Design review of the part built by this model. Coordinates are the model's own, in mm. A direction names the side the tool comes from. Round coordinates to 2 decimals unless told otherwise and drop trailing zeros. Return JSON: item names as keys, results as strings. Group by question number.
(1) We need section A-A, the plane z = 2.05. Give the number of separate pieces and of enclosed holes in the cut face, and give its area (3 significant figures).
(2) For faces 1 (the flat face through (2.533, -12.053, 1.479)), 2 (the flat face through (-2.533, 12.053, 1.479)), 3 (the cylindrical face through (-8.21, -8.05, 1.48)), 4 (the cylindrical face through (-11.13, 9.53, 1.48)), list the 3-axis set-ups (+Z, -Z, +X, -X, +Y, -Y) from which the entire face can be reached by the end or side of a thin tool; tool diameter is ignored.
(3) The part is to be moulded in two halves that separate along Y. For faces 5 (the cylindrical face through (6.02, -9.8, 1.48)), 6 (the cylindrical face through (8.636, 13.469, 1.479)), 7 (the flat face through (-5.354, -11.117, 1.479)), say which applies: pulls with the +Y half, pulls with the -Y half, needs draft (parallel to the pull), parting line crosses it, or undercut.
(4) Clearance check with flat-ended pins moving along their axes: pin 1 (1.3 mm diameter, centred on y = -12.5, z = 1.5, fed in from +X); pin 2 (1.3 mm diameter, centred on y = 12.5, z = 1.5, fed in from -X). State where each tip first meets the part, or that it passes through.
(5) Wall thickness on L1, parallel to X at y = -12, z = 1.5; L2, parallel to Y at x = 13.5, z = 1.4; L3, parallel to X at y = 13, z = 2.45: over which ranges is each line inside the solid? List them lowest first. Write a range as [from, to].
from build123d import *

# Parameters (mm, degrees)
BOSS_EXTRU_1_DEPTH           = 3
R_P_TITION_CIRCULAIRE2_COUNT = 14
ESQUISSE5_R                  = 11.5
BOSS_EXTRU_2_DEPTH           = 3
ESQUISSE6_R                  = 3
ESQUISSE6_R_2                = 1.75
ENL_V_MAT_EXTRU_1_DEPTH      = 4


with BuildPart() as part:
    # Esquisse4 → Boss.-Extru.1 (new body)
    with BuildSketch(Plane.XY):
        with BuildLine():
            Line((0, 13.155696691), (0, 11.5))
            ThreePointArc((0, 11.5), (1.385979557, 11.416175396), (2.751754038, 11.165923594))
            Line((2.751754038, 11.165923594), (3.147934042, 12.773522094))
            ThreePointArc((3.147934042, 12.773522094), (3.010357566, 14.324173734), (2.517223611, 15.800746352))
            ThreePointArc((2.517223611, 15.800746352), (1.928319383, 15.883374464), (1.336751397, 15.944061456))
            ThreePointArc((1.336751397, 15.944061456), (0.504624377, 14.628382005), (0, 13.155696691))
        make_face()
    extrude(amount=BOSS_EXTRU_1_DEPTH)


with BuildPart() as r_p_tition_circulaire2_1:
    # R_p_tition circulaire2: pattern copy
    add(part.part.rotate(Axis((0, 0, 0), (0, 0, 1)), 1 * 360 / R_P_TITION_CIRCULAIRE2_COUNT))


with BuildPart() as r_p_tition_circulaire2_2:
    # R_p_tition circulaire2: pattern copy
    add(part.part.rotate(Axis((0, 0, 0), (0, 0, 1)), 2 * 360 / R_P_TITION_CIRCULAIRE2_COUNT))


with BuildPart() as r_p_tition_circulaire2_3:
    # R_p_tition circulaire2: pattern copy
    add(part.part.rotate(Axis((0, 0, 0), (0, 0, 1)), 3 * 360 / R_P_TITION_CIRCULAIRE2_COUNT))


with BuildPart() as r_p_tition_circulaire2_4:
    # R_p_tition circulaire2: pattern copy
    add(part.part.rotate(Axis((0, 0, 0), (0, 0, 1)), 4 * 360 / R_P_TITION_CIRCULAIRE2_COUNT))


with BuildPart() as r_p_tition_circulaire2_5:
    # R_p_tition circulaire2: pattern copy
    add(part.part.rotate(Axis((0, 0, 0), (0, 0, 1)), 5 * 360 / R_P_TITION_CIRCULAIRE2_COUNT))


with BuildPart() as r_p_tition_circulaire2_6:
    # R_p_tition circulaire2: pattern copy
    add(part.part.rotate(Axis((0, 0, 0), (0, 0, 1)), 6 * 360 / R_P_TITION_CIRCULAIRE2_COUNT))


with BuildPart() as r_p_tition_circulaire2_7:
    # R_p_tition circulaire2: pattern copy
    add(part.part.rotate(Axis((0, 0, 0), (0, 0, 1)), 7 * 360 / R_P_TITION_CIRCULAIRE2_COUNT))


with BuildPart() as r_p_tition_circulaire2_8:
    # R_p_tition circulaire2: pattern copy
    add(part.part.rotate(Axis((0, 0, 0), (0, 0, 1)), 8 * 360 / R_P_TITION_CIRCULAIRE2_COUNT))


with BuildPart() as r_p_tition_circulaire2_9:
    # R_p_tition circulaire2: pattern copy
    add(part.part.rotate(Axis((0, 0, 0), (0, 0, 1)), 9 * 360 / R_P_TITION_CIRCULAIRE2_COUNT))


with BuildPart() as r_p_tition_circulaire2_10:
    # R_p_tition circulaire2: pattern copy
    add(part.part.rotate(Axis((0, 0, 0), (0, 0, 1)), 10 * 360 / R_P_TITION_CIRCULAIRE2_COUNT))


with BuildPart() as r_p_tition_circulaire2_11:
    # R_p_tition circulaire2: pattern copy
    add(part.part.rotate(Axis((0, 0, 0), (0, 0, 1)), 11 * 360 / R_P_TITION_CIRCULAIRE2_COUNT))


with BuildPart() as r_p_tition_circulaire2_12:
    # R_p_tition circulaire2: pattern copy
    add(part.part.rotate(Axis((0, 0, 0), (0, 0, 1)), 12 * 360 / R_P_TITION_CIRCULAIRE2_COUNT))


with BuildPart() as r_p_tition_circulaire2_13:
    # R_p_tition circulaire2: pattern copy
    add(part.part.rotate(Axis((0, 0, 0), (0, 0, 1)), 13 * 360 / R_P_TITION_CIRCULAIRE2_COUNT))


with BuildPart() as part_1:
    add(part.part)

    add(r_p_tition_circulaire2_1.part)  # Boss.-Extru.2 merges R_p_tition circulaire2_1

    add(r_p_tition_circulaire2_2.part)  # Boss.-Extru.2 merges R_p_tition circulaire2_2

    add(r_p_tition_circulaire2_3.part)  # Boss.-Extru.2 merges R_p_tition circulaire2_3

    add(r_p_tition_circulaire2_4.part)  # Boss.-Extru.2 merges R_p_tition circulaire2_4

    add(r_p_tition_circulaire2_5.part)  # Boss.-Extru.2 merges R_p_tition circulaire2_5

    add(r_p_tition_circulaire2_6.part)  # Boss.-Extru.2 merges R_p_tition circulaire2_6

    add(r_p_tition_circulaire2_7.part)  # Boss.-Extru.2 merges R_p_tition circulaire2_7

    add(r_p_tition_circulaire2_8.part)  # Boss.-Extru.2 merges R_p_tition circulaire2_8

    add(r_p_tition_circulaire2_9.part)  # Boss.-Extru.2 merges R_p_tition circulaire2_9

    add(r_p_tition_circulaire2_10.part)  # Boss.-Extru.2 merges R_p_tition circulaire2_10

    add(r_p_tition_circulaire2_11.part)  # Boss.-Extru.2 merges R_p_tition circulaire2_11

    add(r_p_tition_circulaire2_12.part)  # Boss.-Extru.2 merges R_p_tition circulaire2_12

    add(r_p_tition_circulaire2_13.part)  # Boss.-Extru.2 merges R_p_tition circulaire2_13
    # Esquisse5 → Boss.-Extru.2 (add)
    with BuildSketch(Plane.XY):
        Circle(ESQUISSE5_R)
    extrude(amount=BOSS_EXTRU_2_DEPTH)

    # Esquisse6 → Enl_v. mat.-Extru.1 (cut, through all)
    with BuildSketch(Plane(origin=(0, 0, 0), x_dir=(-1, 0, 0), z_dir=(0, 0, -1))):
        Circle(ESQUISSE6_R)
        with Locations((0, 7)):
            Circle(ESQUISSE6_R_2)
        with Locations((7, 0)):
            Circle(ESQUISSE6_R_2)
        with Locations((0, -7)):
            Circle(ESQUISSE6_R_2)
        with Locations((-7, 0)):
            Circle(ESQUISSE6_R_2)
    extrude(amount=-ENL_V_MAT_EXTRU_1_DEPTH, mode=Mode.SUBTRACT)


solid = part_1.part
Solutions:
{
 "1": {"separate pieces": "1", "enclosed holes": "5", "area": "515 mm^2"},
 "2": {"face 1": "+Z, -Z, -Y", "face 2": "+Z, -Z, +Y", "face 3": "+Z, -Z", "face 4": "+Z, -Z, -X"},
 "3": {"face 5": "undercut", "face 6": "pulls with the +Y half", "face 7": "pulls with the -Y half"},
 "4": {"pin 1": "x = 5.89", "pin 2": "x = -5.89"},
 "5": {"L1": "[-9.01, -5.83], [-2.96, 0], [2.52, 5.74]", "L2": "[-6.12, -3.29], [-0.15, 2.9], [7.15, 8.59]", "L3": "[-5.88, -2.76], [0, 3.15], [6.85, 9.12]"}
}
